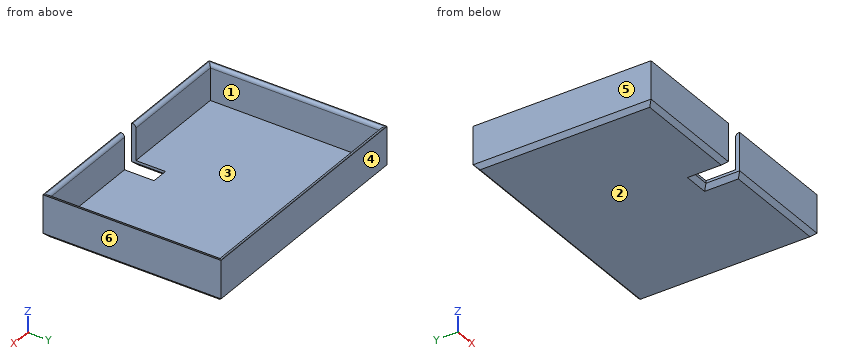
from build123d import *

# Parameters (mm, degrees)
F0_W     = 184.658
F0_H     = 133.858
F1_DEPTH = 5.08
F2_W     = 184.658
F2_H     = 133.858
F2_W_2   = 178.308
F2_H_2   = 127.508
F3_DEPTH = 31.75
F4_W     = 12.7
F4_H     = 31.75
F5_DEPTH = 25.4
F6_SIZE2 = 3.175
F6_SIZE  = 3.175
F7_R     = 2.54


with BuildPart() as f1:
    # F0 (on Top) → F1 (new body)
    with BuildSketch(Plane.XY):
        Rectangle(F0_W, F0_H)
    extrude(amount=F1_DEPTH)

    # F2 (on Top) → F3 (join)
    with BuildSketch(Plane.XY):
        Rectangle(F2_W, F2_H)
        Rectangle(F2_W_2, F2_H_2, mode=Mode.SUBTRACT)
    extrude(amount=F3_DEPTH)

    # F4 (on face) → F5 (cut)
    with BuildSketch(Plane.XZ.offset(66.929)):
        with Locations((0, 15.875)):
            Rectangle(F4_W, F4_H)
    extrude(amount=-F5_DEPTH, mode=Mode.SUBTRACT)

    # F6
    f6_edges = [f1.edges().sort_by_distance(p)[0] for p in [
        (49.3395, -66.929, 0),
        (6.35, -54.229, 0),
        (0, -41.529, 0),
        (-6.35, -54.229, 0),
        (-49.3395, -66.929, 0),
        (-92.329, 0, 0),
        (0, 66.929, 0),
        (92.329, 0, 0),
    ]]
    chamfer(f6_edges, length=F6_SIZE, length2=F6_SIZE2)

    # F7
    f7_edges = [f1.edges().sort_by_distance(p)[0] for p in [
        (47.752, -63.754, 31.75),
        (-47.752, -63.754, 31.75),
        (89.154, 0, 31.75),
        (-89.154, 0, 31.75),
        (0, 63.754, 31.75),
    ]]
    fillet(f7_edges, radius=F7_R)


solid = f1.part
Verification items for the finished model (mm, model axes). Face numbers are marked on the shaded views. A direction names the side the tool comes from. Round coordinates to 2 decimals unless told otherwise and drop trailing zeros. Loops run counter-clockwise (first coordinate to the right, second up) from the corner with the lowest first, then second, coordinate; pieces in that order, holes last. Notation, with made-up numbers: (27.25, 67.5) - (67.25, 67.5) arc R30 cw to (67.25, 101.5) - close; hole circle Ø7 at (48.25, 22.5). An arc over 180 degrees is marked (long way). Answer in a Markdown table with one row per item. Add a question column.
Q1. Material ranges on line 1 (X direction, y = 33, z = 18.5); line 2 (Y direction, x = 24.5, z = 6); line 3 (Z direction, x = 61.5, y = 19.5), recorded low to high.
Q2. Section check B-B on x = 44. Enter the section's corners in (y, z) (3 decimals).
Q3. Tool access check on the marked faces 1 and 2. Record the directions out of +Z, -Z, +X, -X, +Y, -Y that give a thin tool (end or side, any length) a straight path to the whole face; none if there is none.
Q4. Release check for a two-part mould opening along X. For the marked faces 3, 4, 5 and 6 record: pulls with the +X half, pulls with the -X half, needs draft (parallel to the pull), parting line crosses it, or undercut.
Q5. Section check C-C on y = -7.5. Enter the section's corners in (x, z) (3 decimals), plus the area to 3 significant figures.
Q6. Gauge pin test, flat ends, axial feed: pin 1 (6 mm diameter, centred on x = -2.5, z = 18, fed in from -Y); pin 2 (6 mm diameter, centred on x = 71, y = -37.5, fed in from +Z); pin 3 (1.5 mm diameter, centred on x = -1.5, z = 3.5, fed in from -Y). Record the tip position at first contact, or that the pin passes through.
Q7. Section check A-A on y = -50. Enter the section's corners in (x, z) (3 decimals).
Found:
| question | item | result |
|---|---|---|
| 1 | line 1 | x = -92.33 to -89.15, 89.15 to 92.33 |
| 1 | line 2 | y = -66.93 to -63.75, 63.75 to 66.93 |
| 1 | line 3 | z = 0 to 5.08 |
| 2 | outline | (-66.929, 3.175) - (-63.754, 0) - (63.754, 0) - (66.929, 3.175) - (66.929, 31.75) - (66.294, 31.75) arc R2.54 ccw to (63.754, 29.21) - (63.754, 5.08) - (-63.754, 5.08) - (-63.754, 29.21) arc R2.54 ccw to (-66.294, 31.75) - (-66.929, 31.75) - close |
| 3 | face 1 | +Z |
| 3 | face 2 | -Z, +X, -X, +Y, -Y |
| 4 | face 3 | undercut |
| 4 | face 4 | needs draft |
| 4 | face 5 | pulls with the -X half |
| 4 | face 6 | pulls with the +X half |
| 5 | outline | (-92.329, 3.175) - (-89.154, 0) - (89.154, 0) - (92.329, 3.175) - (92.329, 31.75) - (91.694, 31.75) arc R2.54 ccw to (89.154, 29.21) - (89.154, 5.08) - (-89.154, 5.08) - (-89.154, 29.21) arc R2.54 ccw to (-91.694, 31.75) - (-92.329, 31.75) - close |
| 5 | area | 1,090 mm² |
| 6 | pin 1 | stops at y = 63.75 |
| 6 | pin 2 | stops at z = 5.08 |
| 6 | pin 3 | stops at y = -41.53 |
| 7 | outline | (-92.329, 3.175) - (-89.154, 0) - (-9.525, 0) - (-6.35, 3.175) - (-6.35, 5.08) - (-89.154, 5.08) - (-89.154, 29.21) arc R2.54 ccw to (-91.694, 31.75) - (-92.329, 31.75) - close; (6.35, 3.175) - (9.525, 0) - (89.154, 0) - (92.329, 3.175) - (92.329, 31.75) - (91.694, 31.75) arc R2.54 ccw to (89.154, 29.21) - (89.154, 5.08) - (6.35, 5.08) - close |
